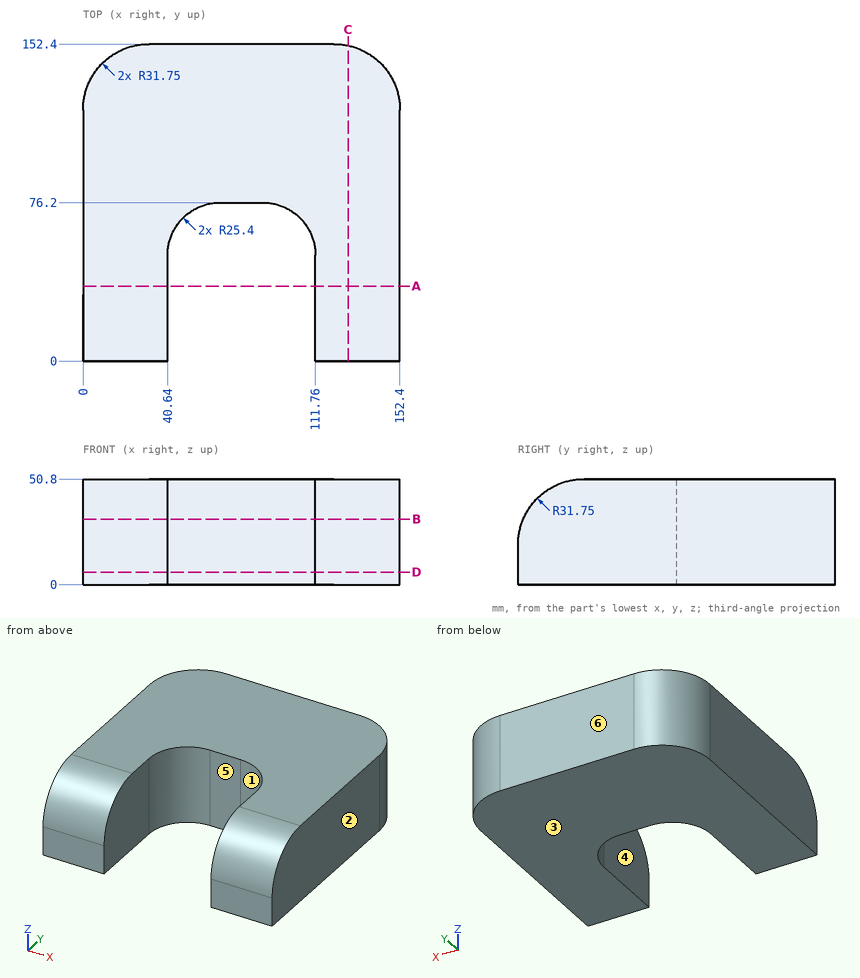
Print and shaded views of the part. All mm, measured from the part's lowest x, y and z. A direction names the side the tool comes from. Coordinates: 2 decimals unless noted, no trailing zeros. Order: outer loops, then holes, each group sorted by start corner. A loop starts at its lowest first (then second) coordinate and runs counter-clockwise, first axis right, second up. Notation, with made-up numbers: M -4.75,-11.75 L 24.25,-11.75 A26 cw 24.25,24.25 Z; hole C 68,83 d10. An arc over 180 degrees is marked long. Write each question's results on one line, items separated by ' | '. Start each with the question number.
Q1. Flat gauge pins, fed straight in: P1, Ø16.5, axis at x = 74, z = 37, coming from the -Y side; P2, Ø1.5, axis at x = 90.5, z = 5.5, coming from the -Y side. Where does each tip first touch, or does it go through?
Q2. Cut at B-B (z = 31.5). List the corners of the cut face in (x, y), then the cut area to 3 significant figures.
Q3. Cut at C-C (x = 127.5). List the corners of the cut face in (y, z).
Q4. Which spindle directions (+Z, -Z, +X, -X, +Y, -Y) get a long thin tool onto all of the face, cutting with end or side? Do the marked faces 5 and 6. Say none if no direction does.
Q5. Drill centre lines: probe 1 along X at (y, z) = (32, 26.5); probe 2 along X at (y, z) = (121.5, 16.5); probe 3 along Y at (x, z) = (32, 19.5). Where is each one in solid material? Low to high. Write a range as from..to.
Q6. Cut at A-A (y = 36). List the corners of the cut face in (x, z).
Q7. Pull direction X, two halves, no side cores. Call the marked faces 1, 2, 3 and 4: +X half, -X half, draft (parallel to the pull), parting line (faces both ways), or undercut.
Q8. Cut at D-D (z = 6). List the corners of the cut face in (x, y), then the cut area to 3 significant figures.
Found:
1) P1: y = 76.2 | P2: y = 75.72
2) outline: M 0,2.54 L 40.64,2.54 L 40.64,50.8 A25.4 cw 66.04,76.2 L 86.36,76.2 A25.4 cw 111.76,50.8 L 111.76,2.54 L 152.4,2.54 L 152.4,120.65 A31.75 ccw 120.65,152.4 L 31.75,152.4 A31.75 ccw 0,120.65 Z | area: 17,400 mm²
3) outline: M 0,0 L 151.65,0 L 151.65,50.8 L 31.75,50.8 A31.75 ccw 0,19.05 Z
4) face 5: +Z, -Z, -Y | face 6: +Z, -Z, +X, -X, +Y
5) probe 1: 0..40.64, 111.76..152.4 | probe 2: 0.01..152.39 | probe 3: 0..152.4
6) outline: M 0,0 L 40.64,0 L 40.64,50.8 L 0,50.8 Z; M 111.76,0 L 152.4,0 L 152.4,50.8 L 111.76,50.8 Z
7) face 1: undercut | face 2: +X half | face 3: draft | face 4: undercut
8) outline: M 0,0 L 40.64,0 L 40.64,50.8 A25.4 cw 66.04,76.2 L 86.36,76.2 A25.4 cw 111.76,50.8 L 111.76,0 L 152.4,0 L 152.4,120.65 A31.75 ccw 120.65,152.4 L 31.75,152.4 A31.75 ccw 0,120.65 Z | area: 17,700 mm²
